```python
from build123d import *

# Parameters (mm, degrees)
SKETCH1_W           = 98.9
SKETCH1_H           = 90
SKETCH1_R           = 4
SKETCH1_R_2         = 25
BOSS_EXTRUDE1_DEPTH = 5
SKETCH2_W           = 5
SKETCH2_H           = 90
BOSS_EXTRUDE2_DEPTH = 10
CHAMFER1_SIZE       = 2


with BuildPart() as part:
    # Sketch1 → Boss-Extrude1 (new body)
    with BuildSketch(Plane(origin=(0, 0, 0), x_dir=(1, 0, 0), z_dir=(0, 1, 0))):
        Rectangle(SKETCH1_W, SKETCH1_H)
        with Locations(Location((37.875, -37.875, 0), (0, 0, 270))):
            Circle(SKETCH1_R, mode=Mode.SUBTRACT)
        with Locations(Location((-37.875, -37.875, 0), (0, 0, 270))):
            Circle(SKETCH1_R, mode=Mode.SUBTRACT)
        with Locations(Location((37.875, 37.875, 0), (0, 0, 270))):
            Circle(SKETCH1_R, mode=Mode.SUBTRACT)
        with Locations(Location((-37.875, 37.875, 0), (0, 0, 270))):
            Circle(SKETCH1_R, mode=Mode.SUBTRACT)
        with Locations(Location((0, 0, 0), (0, 0, 270))):
            Circle(SKETCH1_R_2, mode=Mode.SUBTRACT)
    extrude(amount=BOSS_EXTRUDE1_DEPTH)

    # Sketch2 → Boss-Extrude2 (add)
    with BuildSketch(Plane.XZ):
        with Locations((-46.95, 0)):
            Rectangle(SKETCH2_W, SKETCH2_H)
        with Locations((46.95, 0)):
            Rectangle(SKETCH2_W, SKETCH2_H)
    extrude(amount=BOSS_EXTRUDE2_DEPTH)

    # Chamfer1
    chamfer1_edges = [part.edges().sort_by_distance(p)[0] for p in [
        (-44.45, -10, 0),
        (44.45, -10, 0),
    ]]
    chamfer(chamfer1_edges, length=CHAMFER1_SIZE)


solid = part.part
```
The listing builds one solid part. Answer for the finished solid, in the listing's coordinates (mm). A direction names the side the tool comes from. Round coordinates to 2 decimals unless told otherwise and drop trailing zeros. Order: outer loops, then holes, each group sorted by start corner. A loop starts at its lowest first (then second) coordinate and runs counter-clockwise, first axis right, second up. Notation, with made-up numbers: (-21, 22) -> (29, 22) arc R8 ccw to (29, 27) -> close; hole circle Ø4 at (87.25, -34). An arc over 180 degrees is marked (long way). Answer as CSV lines item,"result".
Q1. Given pin 1 (12 mm diameter, centred on x = -20, z = -6.5, fed in from -Y); pin 2 (13 mm diameter, centred on x = -37.875, z = -37.875, fed in from +Y), each flat-ended and moving along its own axis, determine where each tip first touches the part or whether it passes through.
Computed values:
pin 1,"stops at y = 0"
pin 2,"stops at y = 5"
Q2. A cutting plane is placed at D-D on z = -27. Determine the outline of the cut face in (x, y).
Computed values:
outline,"(-49.45, -10) -> (-46.45, -10) -> (-44.45, -8) -> (-44.45, 0) -> (44.45, 0) -> (44.45, -8) -> (46.45, -10) -> (49.45, -10) -> (49.45, 5) -> (-49.45, 5) -> close"
Q3. Consider line 1 (X direction, y = -3.5, z = 34); line 2 (Z direction, x = 39.5, y = 3); line 3 (X direction, y = 1.85, z = 0). Determine where each line is inside the solid, lowest interval first. Write a range as from..to.
Computed values:
line 1,"x = -49.45..-44.45, 44.45..49.45"
line 2,"z = -45..-41.53, -34.22..34.22, 41.53..45"
line 3,"x = -49.45..-25, 25..49.45"
Q4. A cutting plane is placed at C-C on x = 0. Determine the outline of the cut face in (y, z).
Computed values:
outline,"(0, -45) -> (5, -45) -> (5, -25) -> (0, -25) -> close; (0, 25) -> (5, 25) -> (5, 45) -> (0, 45) -> close"
Q5. Which of the six approach directions +Z, -Z, +X, -X, +Y, -Y give full straight-line access (tool end or side, diameter ignored) to faces 1 (the cylindrical face through (41.84, 2.46, 37.35)), 2 (the flat face through (44.45, -4, -1))?
Computed values:
face 1,"+Y, -Y"
face 2,"+Z, -Z, -Y"
Q6. A cutting plane is placed at B-B on y = -2. Determine the outline of the cut face in (x, z), plus the area to 3 significant figures.
Computed values:
outline,"(-49.45, -45) -> (-44.45, -45) -> (-44.45, 45) -> (-49.45, 45) -> close; (44.45, -45) -> (49.45, -45) -> (49.45, 45) -> (44.45, 45) -> close"
area,"900 mm^2"
Q7. A cutting plane is placed at A-A on z = 0. Determine the outline of the cut face in (x, y), plus the area to 4 significant figures.
Computed values:
outline,"(-49.45, -10) -> (-46.45, -10) -> (-44.45, -8) -> (-44.45, 0) -> (-25, 0) -> (-25, 5) -> (-49.45, 5) -> close; (25, 0) -> (44.45, 0) -> (44.45, -8) -> (46.45, -10) -> (49.45, -10) -> (49.45, 5) -> (25, 5) -> close"
area,"340.5 mm^2"
Q8. For a pull along X with two mould halves and no side action, classify faces 3 (the cylindrical face through (7.509, 2.465, 23.846)), 4 (the flat face through (-48, -10, 1)), 5 (the flat face through (-49.45, -2, -1)) as +X half, -X half, draft (parallel to the pull), parting line (faces both ways), or undercut.
Computed values:
face 3,"undercut"
face 4,"draft"
face 5,"-X half"
